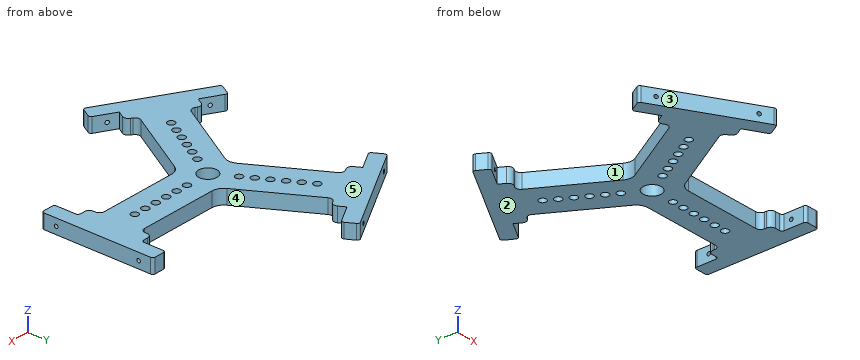
```python
from build123d import *

# Parameters (mm, degrees)
ESQUISSE1_R                  = 3
ESQUISSE1_R_2                = 7.55
BOSS_EXTRU_1_DEPTH           = 6
ESQUISSE2_R                  = 1.5
ENL_V_MAT_EXTRU_1_DEPTH      = 219.511470169
R_P_TITION_CIRCULAIRE1_COUNT = 3


with BuildPart() as part:
    # Esquisse1 → Boss.-Extru.1 (new, symmetric)
    with BuildSketch(Plane.XY):
        with BuildLine():
            Line((93.969262079, 44.202014333), (93.969262079, 28.202014333))
            ThreePointArc((93.969262079, 28.202014333), (93.383475641, 26.78780077), (91.969262079, 26.202014333))
            Line((91.969262079, 26.202014333), (87.969262079, 26.202014333))
            ThreePointArc((87.969262079, 26.202014333), (85.140834954, 25.030441457), (83.969262079, 22.202014333))
            Line((83.969262079, 22.202014333), (83.969262079, 20.710100717))
            ThreePointArc((83.969262079, 20.710100717), (82.797689203, 17.881673592), (79.969262079, 16.710100717))
            Line((79.969262079, 16.710100717), (15.421083839, 16.710100717))
            ThreePointArc((15.421083839, 16.710100717), (10.421083839, 18.049846679), (6.760829801, 21.710100717))
            Line((6.760829801, 21.710100717), (-25.513259319, 77.61046284))
            ThreePointArc((-25.513259319, 77.61046284), (-25.912861009, 80.645739021), (-24.049157704, 83.074564455))
            Line((-24.049157704, 83.074564455), (-22.757122612, 83.820521263))
            ThreePointArc((-22.757122612, 83.820521263), (-20.893419307, 86.249346698), (-21.293020997, 89.284622879))
            Line((-21.293020997, 89.284622879), (-24.293020997, 94.480775301))
            Line((-24.293020997, 94.480775301), (-8.704563729, 103.480775301))
            ThreePointArc((-8.704563729, 103.480775301), (-7.772712076, 104.695188019), (-7.972512921, 106.212826109))
            Line((-7.972512921, 106.212826109), (-11.972512921, 113.141029339))
            ThreePointArc((-11.972512921, 113.141029339), (-13.186925639, 114.072880992), (-14.704563729, 113.873080147))
            Line((-14.704563729, 113.873080147), (-91.26469835, 69.671065814))
            ThreePointArc((-91.26469835, 69.671065814), (-92.196550002, 68.456653097), (-91.996749157, 66.939015006))
            Line((-91.996749157, 66.939015006), (-87.996749157, 60.010811776))
            ThreePointArc((-87.996749157, 60.010811776), (-86.78233644, 59.078960124), (-85.26469835, 59.278760969))
            Line((-85.26469835, 59.278760969), (-69.676241082, 68.278760969))
            Line((-69.676241082, 68.278760969), (-66.676241082, 63.082608546))
            ThreePointArc((-66.676241082, 63.082608546), (-64.247415647, 61.218905241), (-61.212139466, 61.618506931))
            Line((-61.212139466, 61.618506931), (-59.920104375, 62.364463739))
            ThreePointArc((-59.920104375, 62.364463739), (-56.884828194, 62.764065429), (-54.45600276, 60.900362124))
            Line((-54.45600276, 60.900362124), (-22.18191364, 5))
            ThreePointArc((-22.18191364, 5), (-20.842167678, 0), (-22.18191364, -5))
            Line((-22.18191364, -5), (-54.45600276, -60.900362124))
            ThreePointArc((-54.45600276, -60.900362124), (-56.884828194, -62.764065429), (-59.920104375, -62.364463739))
            Line((-59.920104375, -62.364463739), (-61.212139466, -61.618506931))
            ThreePointArc((-61.212139466, -61.618506931), (-64.247415647, -61.218905241), (-66.676241082, -63.082608546))
            Line((-66.676241082, -63.082608546), (-69.676241082, -68.278760969))
            Line((-69.676241082, -68.278760969), (-85.26469835, -59.278760969))
            ThreePointArc((-85.26469835, -59.278760969), (-86.78233644, -59.078960124), (-87.996749157, -60.010811776))
            Line((-87.996749157, -60.010811776), (-91.996749157, -66.939015007))
            ThreePointArc((-91.996749157, -66.939015007), (-92.196550002, -68.456653097), (-91.26469835, -69.671065814))
            Line((-91.26469835, -69.671065814), (-14.704563729, -113.873080147))
            ThreePointArc((-14.704563729, -113.873080147), (-13.186925639, -114.072880992), (-11.972512921, -113.141029339))
            Line((-11.972512921, -113.141029339), (-7.972512921, -106.212826109))
            ThreePointArc((-7.972512921, -106.212826109), (-7.772712076, -104.695188019), (-8.704563729, -103.480775301))
            Line((-8.704563729, -103.480775301), (-24.293020997, -94.480775301))
            Line((-24.293020997, -94.480775301), (-21.293020997, -89.284622879))
            ThreePointArc((-21.293020997, -89.284622879), (-20.893419307, -86.249346698), (-22.757122612, -83.820521263))
            Line((-22.757122612, -83.820521263), (-24.049157704, -83.074564455))
            ThreePointArc((-24.049157704, -83.074564455), (-25.912861009, -80.645739021), (-25.513259319, -77.61046284))
            Line((-25.513259319, -77.61046284), (6.760829801, -21.710100717))
            ThreePointArc((6.760829801, -21.710100717), (10.421083839, -18.049846679), (15.421083839, -16.710100717))
            Line((15.421083839, -16.710100717), (79.969262079, -16.710100717))
            ThreePointArc((79.969262079, -16.710100717), (82.797689203, -17.881673592), (83.969262079, -20.710100717))
            Line((83.969262079, -20.710100717), (83.969262079, -22.202014333))
            ThreePointArc((83.969262079, -22.202014333), (85.140834954, -25.030441457), (87.969262079, -26.202014333))
            Line((87.969262079, -26.202014333), (91.969262079, -26.202014333))
            ThreePointArc((91.969262079, -26.202014333), (93.383475641, -26.78780077), (93.969262079, -28.202014333))
            Line((93.969262079, -28.202014333), (93.969262079, -44.202014333))
            ThreePointArc((93.969262079, -44.202014333), (94.555048516, -45.616227895), (95.969262079, -46.202014333))
            Line((95.969262079, -46.202014333), (103.969262079, -46.202014333))
            ThreePointArc((103.969262079, -46.202014333), (105.383475641, -45.616227895), (105.969262079, -44.202014333))
            Line((105.969262079, -44.202014333), (105.969262079, 44.202014333))
            ThreePointArc((105.969262079, 44.202014333), (105.383475641, 45.616227895), (103.969262079, 46.202014333))
            Line((103.969262079, 46.202014333), (95.969262079, 46.202014333))
            ThreePointArc((95.969262079, 46.202014333), (94.555048516, 45.616227895), (93.969262079, 44.202014333))
        make_face()
        with Locations((-35, -60.621778265)):
            Circle(ESQUISSE1_R, mode=Mode.SUBTRACT)
        with Locations((-30, -51.961524227)):
            Circle(ESQUISSE1_R, mode=Mode.SUBTRACT)
        with Locations((-25, -43.301270189)):
            Circle(ESQUISSE1_R, mode=Mode.SUBTRACT)
        with Locations((-20, -34.641016151)):
            Circle(ESQUISSE1_R, mode=Mode.SUBTRACT)
        with Locations((-15, -25.980762114)):
            Circle(ESQUISSE1_R, mode=Mode.SUBTRACT)
        with Locations((-10, -17.320508076)):
            Circle(ESQUISSE1_R, mode=Mode.SUBTRACT)
        with Locations((-10, 17.320508076)):
            Circle(ESQUISSE1_R, mode=Mode.SUBTRACT)
        with Locations((-15, 25.980762114)):
            Circle(ESQUISSE1_R, mode=Mode.SUBTRACT)
        with Locations((-20, 34.641016151)):
            Circle(ESQUISSE1_R, mode=Mode.SUBTRACT)
        with Locations((-25, 43.301270189)):
            Circle(ESQUISSE1_R, mode=Mode.SUBTRACT)
        with Locations((-30, 51.961524227)):
            Circle(ESQUISSE1_R, mode=Mode.SUBTRACT)
        with Locations((-35, 60.621778265)):
            Circle(ESQUISSE1_R, mode=Mode.SUBTRACT)
        with Locations((20, 0)):
            Circle(ESQUISSE1_R, mode=Mode.SUBTRACT)
        with Locations((30, 0)):
            Circle(ESQUISSE1_R, mode=Mode.SUBTRACT)
        with Locations((40, 0)):
            Circle(ESQUISSE1_R, mode=Mode.SUBTRACT)
        with Locations((50, 0)):
            Circle(ESQUISSE1_R, mode=Mode.SUBTRACT)
        with Locations((60, 0)):
            Circle(ESQUISSE1_R, mode=Mode.SUBTRACT)
        with Locations((70, 0)):
            Circle(ESQUISSE1_R, mode=Mode.SUBTRACT)
        Circle(ESQUISSE1_R_2, mode=Mode.SUBTRACT)
    extrude(amount=BOSS_EXTRU_1_DEPTH, both=True)

    # Esquisse2 → Enlèv. mat.-Extru.1 (cut, through all)
    with BuildSketch(Plane.ZY.offset(-93.969262079)):
        with Locations((0, 34.202014333)):
            Circle(ESQUISSE2_R)
        with Locations((0, -34.202014333)):
            Circle(ESQUISSE2_R)
    enl_v_mat_extru_1 = extrude(amount=-ENL_V_MAT_EXTRU_1_DEPTH, mode=Mode.SUBTRACT)

    # Répétition circulaire1: Enlèv. mat.-Extru.1 ×3 about axis
    r_p_tition_circulaire1_axis = Axis((0, 0, 6), (0, 0, -1))
    for i in range(1, R_P_TITION_CIRCULAIRE1_COUNT):
        add(enl_v_mat_extru_1.rotate(r_p_tition_circulaire1_axis, i * 360 / R_P_TITION_CIRCULAIRE1_COUNT), mode=Mode.SUBTRACT)


solid = part.part
```
Geometry check sheet. Reference: the model listing, model coordinates, mm. Face numbers are marked on the shaded views. A direction names the side the tool comes from. Give positions to 0.01 mm unless a question says otherwise; leave off trailing zeros. Loops run counter-clockwise (first coordinate to the right, second up) from the corner with the lowest first, then second, coordinate; pieces in that order, holes last. Notation, with made-up numbers: M -33.75,49.5 L 24.25,49.5 A19 cw 24.25,61.5 Z; hole C 13.5,16 d11. An arc over 180 degrees is marked long. Write item = value, one per line.
(1) Release check for a two-part mould opening along Y. For the marked faces 1, 2 and 3 record: released by +Y, released by -Y, zero draft, split by the parting line, or undercut.
Answer below:
face_1 = undercut
face_2 = zero draft
face_3 = released by -Y
(2) Material ranges on line 1 (Y direction, x = 50, z = 0.25); line 2 (X direction, y = -18, z = -4.75); line 3 (Y direction, x = -14, z = 3.5), recorded low to high. Write a range as [from, to].
Answer below:
line_1 = [-16.71, -3], [3, 16.71]
line_2 = [-29.69, -12.92], [-7.08, 10.51], [82.91, 105.97]
line_3 = [-114.12, -100.42], [-57.67, -28.81], [-23.15, 23.15], [28.81, 57.67], [100.42, 114.12]
(3) Tool access check on the marked faces 4 and 5. Record the directions out of +Z, -Z, +X, -X, +Y, -Y that give a thin tool (end or side, any length) a straight path to the whole face; none if there is none.
Answer below:
face_4 = +Z, -Z
face_5 = +Z, +X, -X, +Y, -Y
(4) Gauge pin test, flat ends, axial feed: pin 1 Ø4.5 at (x, z) = (89, -2) entering from +Y; pin 2 Ø1.2 at (y, z) = (-21.5, -1) entering from -X; pin 3 Ø4 at (y, z) = (35, -4) entering from -X. Record the tip position at first contact, or that the pin passes through.
Answer below:
pin_1 = 26.2
pin_2 = -32.05
pin_3 = -40.66
(5) Sectioned sample at A-A, the plane x = 20. Record the cut outline in (y, z), plus the area to 3 significant figures.
Answer below:
outline = M -16.71,-6 L -3,-6 L -3,6 L -16.71,6 Z; M 3,-6 L 16.71,-6 L 16.71,6 L 3,6 Z
area = 329 mm2
